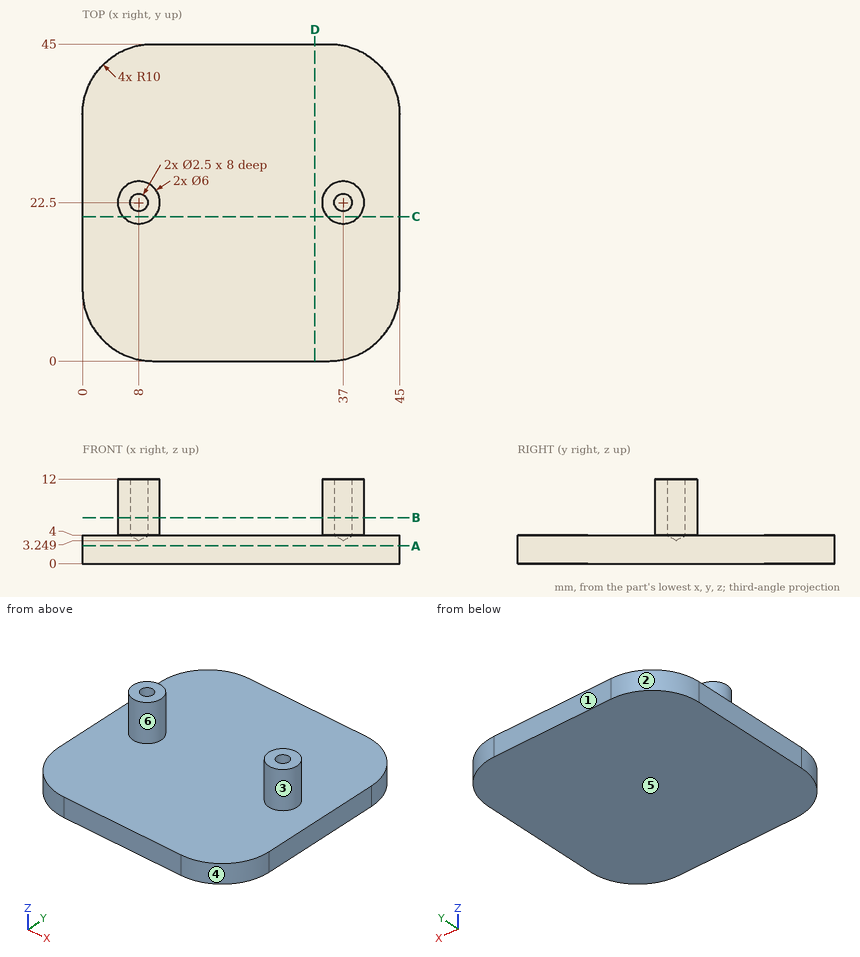
Part print with two shaded views. Sizes in mm from the minimum x, y, z corner. A direction names the side the tool comes from. Coordinates: 2 decimals unless noted, no trailing zeros. Order: outer loops, then holes, each group sorted by start corner. A loop starts at its lowest first (then second) coordinate and runs counter-clockwise, first axis right, second up.
(1) Saw through at A-A, the plane z = 2.5. Write the cut outline in (x, y).
Solution:
outline: (0, 10) arc R10 ccw to (10, 0) - (35, 0) arc R10 ccw to (45, 10) - (45, 35) arc R10 ccw to (35, 45) - (10, 45) arc R10 ccw to (0, 35) - close
(2) Pin check, flat tip, straight feed: pin 1 Ø5 at (x, y) = (9, 33) entering from +Z. Stop position of the tip, or through.
Solution:
pin 1: stops at z = 4
(3) Mould opens along X. For the marked faces 1, 2, 3 and 4 say: released by +X, released by -X, zero draft, split by the parting line, or undercut.
Solution:
face 1: zero draft
face 2: released by -X
face 3: undercut
face 4: released by +X
(4) Saw through at C-C, the plane y = 20.5. Write the cut outline in (x, z).
Solution:
outline: (0, 0) - (45, 0) - (45, 4) - (39.24, 4) - (39.24, 12) - (34.76, 12) - (34.76, 4) - (10.24, 4) - (10.24, 12) - (5.76, 12) - (5.76, 4) - (0, 4) - close
(5) Which spindle directions (+Z, -Z, +X, -X, +Y, -Y) get a long thin tool onto all of the face, cutting with end or side? Do the marked faces 5 and 6. Say none if no direction does.
Solution:
face 5: -Z, +X, -X, +Y, -Y
face 6: +Z
(6) Drill centre lines: L1, parallel to Y at x = 37, z = 7.25; L2, parallel to Z at x = 16, y = 37; L3, parallel to Y at x = 8.5, z = 2.75. Where is each one in solid material? Low to high.
Solution:
L1: y = 19.5 to 21.25, 23.75 to 25.5
L2: z = 0 to 4
L3: y = 0.11 to 44.89
(7) Saw through at B-B, the plane z = 6.5. Write the cut outline in (x, y), and give its area (3 significant figures).
Solution:
outline: circle Ø6 at (8, 22.5); circle Ø6 at (37, 22.5); hole circle Ø2.5 at (8, 22.5); hole circle Ø2.5 at (37, 22.5)
area: 46.7 mm2
(8) Saw through at D-D, the plane x = 33. Write the cut outline in (y, z).
Solution:
outline: (0, 0) - (45, 0) - (45, 4) - (0, 4) - close
